Design review of the part built by this model. Coordinates are the model's own, in mm. Face numbers are marked on the shaded views. A direction names the side the tool comes from. Give positions to 0.01 mm unless a question says otherwise; leave off trailing zeros. Order: outer loops, then holes, each group sorted by start corner. A loop starts at its lowest first (then second) coordinate and runs counter-clockwise, first axis right, second up. Notation, with made-up numbers: (-10, 67.25) -> (15, 67.25) arc R19 cw to (15, 98.25) -> close; hole circle Ø10 at (76.25, 33.25). An arc over 180 degrees is marked (long way). Return JSON: item names as keys, results as strings.
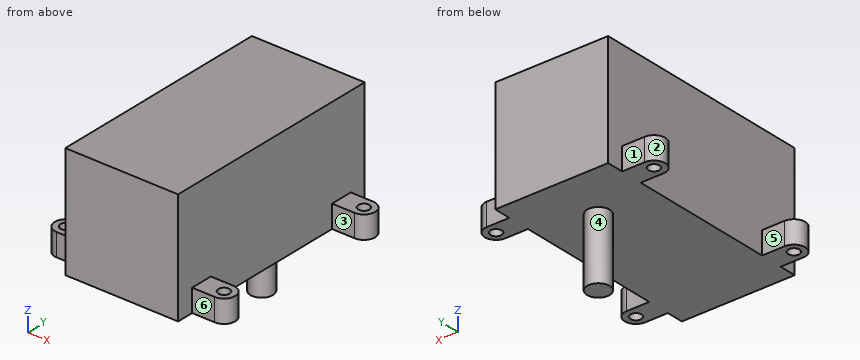
```python
from build123d import *

# Parameters (mm, degrees)
SKETCH1_W           = 100
SKETCH1_H           = 50
BOSS_EXTRUDE1_DEPTH = 50
SKETCH2_R           = 2.5
BOSS_EXTRUDE2_DEPTH = 10
SKETCH3_R           = 5
BOSS_EXTRUDE3_DEPTH = 30


with BuildPart() as part:
    # Sketch1 → Boss-Extrude1 (new body)
    with BuildSketch(Plane(origin=(0, 0, 0), x_dir=(0, 1, 0), z_dir=(0, 0, 1))):
        with Locations((45, -21.706161137)):
            Rectangle(SKETCH1_W, SKETCH1_H)
    extrude(amount=BOSS_EXTRUDE1_DEPTH)

    # Sketch2 → Boss-Extrude2 (add)
    # profile 1 of 4: a face of its own
    with BuildSketch(Plane(origin=(0, 0, 0), x_dir=(1, 0, 0), z_dir=(0, 0, -1))):
        with BuildLine():
            Line((-3.293838863, -2.5), (-13.293838863, -2.5))
            ThreePointArc((-13.293838863, -2.5), (-18.293838863, -7.5), (-13.293838863, -12.5))
            Line((-13.293838863, -12.5), (-3.293838863, -12.5))
            Line((-3.293838863, -12.5), (-3.293838863, -2.5))
        make_face()
        with Locations(Location((-13.293838863, -7.5, 0), (0, 0, 180))):
            Circle(SKETCH2_R, mode=Mode.SUBTRACT)
    # profile 2 of 4: a face of its own
    with BuildSketch(Plane(origin=(0, 0, 0), x_dir=(1, 0, 0), z_dir=(0, 0, -1))):
        with BuildLine():
            Line((-3.293838863, -77.5), (-3.293838863, -87.5))
            Line((-3.293838863, -87.5), (-13.293838863, -87.5))
            ThreePointArc((-13.293838863, -87.5), (-18.293838863, -82.5), (-13.293838863, -77.5))
            Line((-13.293838863, -77.5), (-3.293838863, -77.5))
        make_face()
        with Locations((-13.293838863, -82.5)):
            Circle(SKETCH2_R, mode=Mode.SUBTRACT)
    # profile 3 of 4: a face of its own
    with BuildSketch(Plane(origin=(0, 0, 0), x_dir=(1, 0, 0), z_dir=(0, 0, -1))):
        with BuildLine():
            Line((46.706161137, -87.5), (56.706161137, -87.5))
            ThreePointArc((56.706161137, -87.5), (61.706161137, -82.5), (56.706161137, -77.5))
            Line((56.706161137, -77.5), (46.706161137, -77.5))
            Line((46.706161137, -77.5), (46.706161137, -87.5))
        make_face()
        with Locations(Location((56.706161137, -82.5, 0), (0, 0, 180))):
            Circle(SKETCH2_R, mode=Mode.SUBTRACT)
    # profile 4 of 4: a face of its own
    with BuildSketch(Plane(origin=(0, 0, 0), x_dir=(1, 0, 0), z_dir=(0, 0, -1))):
        with BuildLine():
            Line((46.706161137, -12.5), (46.706161137, -2.5))
            Line((46.706161137, -2.5), (56.706161137, -2.5))
            ThreePointArc((56.706161137, -2.5), (61.706161137, -7.5), (56.706161137, -12.5))
            Line((56.706161137, -12.5), (46.706161137, -12.5))
        make_face()
        with Locations((56.706161137, -7.5)):
            Circle(SKETCH2_R, mode=Mode.SUBTRACT)
    extrude(amount=-BOSS_EXTRUDE2_DEPTH)

    # Sketch3 → Boss-Extrude3 (add)
    with BuildSketch(Plane(origin=(0, 0, 0), x_dir=(1, 0, 0), z_dir=(0, 0, -1))):
        with Locations(Location((21.706161137, -70, 0), (0, 0, 180))):
            Circle(SKETCH3_R)
    extrude(amount=BOSS_EXTRUDE3_DEPTH)


solid = part.part
```
Item 1: Add section B-B (y = 7.5). Give the boundary of the cut face in (x, z), plus the area to 3 significant figures.
Result set:
{"outline": "(-18.29, 0) -> (-15.79, 0) -> (-15.79, 10) -> (-18.29, 10) -> close; (-10.79, 0) -> (54.21, 0) -> (54.21, 10) -> (46.71, 10) -> (46.71, 50) -> (-3.29, 50) -> (-3.29, 10) -> (-10.79, 10) -> close; (59.21, 0) -> (61.71, 0) -> (61.71, 10) -> (59.21, 10) -> close", "area": "2,700 mm^2"}
Item 2: Wall thickness on L1, parallel to X at y = 82, z = 6; L2, parallel to Z at x = 38.5, y = 36.5; L3, parallel to X at y = 89, z = 15.5: over which ranges is each line inside the solid? List them lowest first. Write a range as [from, to].
Result set:
{"L1": "x = [-18.27, -15.74], [-10.84, 54.26], [59.16, 61.68]", "L2": "z = [0, 50]", "L3": "x = [-3.29, 46.71]"}
Item 3: Add section A-A (x = -9). Give the boundary of the cut face in (y, z).
Result set:
{"outline": "(2.5, 0) -> (12.5, 0) -> (12.5, 10) -> (2.5, 10) -> close; (77.5, 0) -> (87.5, 0) -> (87.5, 10) -> (77.5, 10) -> close"}
Item 4: For pin 1 (5 mm diameter, centred on x = -8.5, y = 84.5, fed in from +Z); pin 2 (6 mm diameter, centred on x = 18.5, z = -17.5, fed in from +Y); pin 3 (3 mm diameter, centred on x = 53, z = 5.5, fed in from +Y), all flat-tipped, find the tip position at first contact; note any pin that passes through.
Result set:
{"pin 1": "stops at z = 10", "pin 2": "stops at y = 75", "pin 3": "stops at y = 87.5"}
Item 5: Add section D-D (z = 38.5). Give the boundary of the cut face in (x, y).
Result set:
{"outline": "(-3.29, -5) -> (46.71, -5) -> (46.71, 95) -> (-3.29, 95) -> close"}
Item 6: Machinability: for the marked faces 1, 2 and 3, which of the approach directions +Z, -Z, +X, -X, +Y, -Y give a long, thin tool a straight path to every point of the face, cutting with its end or side? Answer none if there is none.
Result set:
{"face 1": "+Z, -Z, -X, +Y", "face 2": "+Z, -Z, -X", "face 3": "+Z, -Z, +X"}
Item 7: Mouldability with a two-part tool opening along Y and no side actions: class the marked faces 4, 5 and 6 as released by +Y, released by -Y, zero draft, split by the parting line, or undercut.
Result set:
{"face 4": "split by the parting line", "face 5": "undercut", "face 6": "released by -Y"}
Item 8: Add section C-C (y = 70). Give the boundary of the cut face in (x, z).
Result set:
{"outline": "(-3.29, 0) -> (16.71, 0) -> (16.71, -30) -> (26.71, -30) -> (26.71, 0) -> (46.71, 0) -> (46.71, 50) -> (-3.29, 50) -> close"}
